from build123d import *

# Parameters (mm, degrees)
SKETCH1_W          = 4
SKETCH1_H          = 0.5
SKETCH6_OUTSIDE_W  = 7.73
SKETCH6_OUTSIDE_H  = 7.48
CUT_EXTRUDE1_DEPTH = 8.809622956
SKETCH7_R          = 1
CUT_EXTRUDE2_DEPTH = 0.5


with BuildPart() as part:
    # Sweep1: sweep along a path in Sketch2
    with BuildLine(Plane(origin=(0, 0, 0), x_dir=(0, 0, -1), z_dir=(1, 0, 0))) as sweep1_path:
        Line((0, 0), (0, -5.609611797))
        ThreePointArc((0, -5.609611797), (0.105897281, -5.917317901), (0.378732187, -6.094683047))
        Line((0.378732187, -6.094683047), (1.695534419, -6.423883605))
        ThreePointArc((1.695534419, -6.423883605), (1.971967014, -6.414126872), (2.200912871, -6.258904554))
        Line((2.200912871, -6.258904554), (3.13411064, -5.139067232))
        ThreePointArc((3.13411064, -5.139067232), (3.220135789, -4.989187664), (3.25, -4.818975032))
        Line((3.25, -4.818975032), (3.25, -3))
    # Sketch1 → Sweep1 (sweep)
    with BuildSketch(Plane(origin=(0, 0, 0), x_dir=(1, 0, 0), z_dir=(0, 1, 0))):
        Rectangle(SKETCH1_W, SKETCH1_H)
    sweep(path=sweep1_path.line)

    # Sketch6 outside → Cut-Extrude1 (cut, through all)
    with BuildSketch(Plane(origin=(0, 0, 0), x_dir=(1, 0, 0), z_dir=(0, 1, 0))):
        with Locations((0, 1.625)):
            Rectangle(SKETCH6_OUTSIDE_W, SKETCH6_OUTSIDE_H)
        Polygon((2, -0.25), (-2, -0.25), (-2, 0.25), (-1, 3), (-1, 3.5), (1, 3.5), (1, 3), (2, 0.25), align=None, mode=Mode.SUBTRACT)
    extrude(amount=-CUT_EXTRUDE1_DEPTH, mode=Mode.SUBTRACT)

    # Sketch7 → Cut-Extrude2 (cut)
    with BuildSketch(Plane.XY.offset(0.25)):
        with Locations((0, -3.5)):
            Circle(SKETCH7_R)
    extrude(amount=-CUT_EXTRUDE2_DEPTH, mode=Mode.SUBTRACT)


solid = part.part
The listing builds one solid part. Answer for the finished solid, in the listing's coordinates (mm). A direction names the side the tool comes from. Round coordinates to 2 decimals unless told otherwise and drop trailing zeros. Order: outer loops, then holes, each group sorted by start corner. A loop starts at its lowest first (then second) coordinate and runs counter-clockwise, first axis right, second up. Notation, with made-up numbers: (19, 4.25) -> (27, 4.25) arc R14 cw to (27, 22.25) -> close; hole circle Ø7 at (65.25, 64). An arc over 180 degrees is marked (long way). Put each result on its own line as item: value.
Q1. Section C-C, the plane y = -5.5 is taken. Write down the section's boundary in (x, z), and give its area (3 significant figures).
Results list:
outline: (-2, -0.25) -> (2, -0.25) -> (2, 0.25) -> (-2, 0.25) -> close; (-1.18, -2.51) -> (-1, -3) -> (-1, -3.16) -> (1, -3.16) -> (1, -3) -> (1.18, -2.51) -> close
area: 3.39 mm^2
Q2. Section D-D, the plane z = 0.05 is taken. Write down the section's boundary in (x, y).
Results list:
outline: (-2, -6.12) -> (2, -6.12) -> (2, 0) -> (-2, 0) -> close; hole circle Ø2 at (0, -3.5)
Q3. This flat-tipped pin is pushed along its axis until it touches: P1, Ø0.9, axis at x = 0, y = -4, coming from the +Z side. Where does it stop, or does it pass through?
Results list:
P1: z = -3
Q4. Section A-A, the plane x = 0 is taken. Write down the section's boundary in (y, z), and give its area (3 significant figures).
Results list:
outline: (-6.67, -1.63) arc R0.75 ccw to (-6.42, -2.39) -> (-5.3, -3.33) arc R0.75 ccw to (-4.82, -3.5) -> (-3, -3.5) -> (-3, -3) -> (-4.82, -3) arc R0.25 cw to (-4.98, -2.94) -> (-6.1, -2.01) arc R0.25 cw to (-6.18, -1.76) -> (-5.85, -0.44) arc R0.25 cw to (-5.61, -0.25) -> (-4.5, -0.25) -> (-4.5, 0.25) -> (-5.61, 0.25) arc R0.75 ccw to (-6.34, -0.32) -> close; (-2.5, -0.25) -> (0, -0.25) -> (0, 0.25) -> (-2.5, 0.25) -> close
area: 4.91 mm^2
Q5. Which of the six approach directions +Z, -Z, +X, -X, +Y, -Y give full straight-line access (tool end or side, diameter ignored) to faces 4 (the flat face through (-0.017, -5.851, -2.866)), 5 (the flat face through (0, -2, -0.25))?
Results list:
face 4: -Z, +X, -X, -Y
face 5: +X, -X, +Y
Q6. Section B-B, the plane y = -3.5 is taken. Write down the section's boundary in (x, z).
Results list:
outline: (-2, -0.25) -> (-1, -0.25) -> (-1, 0.25) -> (-2, 0.25) -> close; (-1, -3.5) -> (1, -3.5) -> (1, -3) -> (-1, -3) -> close; (1, -0.25) -> (2, -0.25) -> (2, 0.25) -> (1, 0.25) -> close
Q7. Consider line 1 along Z through (x, y) = (-0.3, -4.5); line 2 along Z through (x, y) = (-0.9, -3.5); line 3 along Y through (x, z) = (0, 0). Determine where each line is inside the solid, lowest interval first.
Results list:
line 1: -3.5 to -3, -0.25 to 0.25
line 2: -3.5 to -3
line 3: -6.17 to -4.5, -2.5 to 0
Q8. Determine the mould class of faces 1 (the cylindrical face through (0.954, -3.2, 0.004)), 2 (the flat face through (-0.028, -6.504, -0.986)), 3 (the flat face through (0.03, -6.02, -1.11)) for opening direction Y: pulls with the +Y half, pulls with the -Y half, needs draft (parallel to the pull), parting line crosses it, or undercut.
Results list:
face 1: undercut
face 2: pulls with the -Y half
face 3: pulls with the +Y half
